Geometry: see drawing. Coordinates: mm, zero at the bounding-box minimum. A direction names the side the tool comes from. Coordinates: 2 decimals unless noted, no trailing zeros. Order: outer loops, then holes, each group sorted by start corner. A loop starts at its lowest first (then second) coordinate and runs counter-clockwise, first axis right, second up.
Item 1: Section A-A on y = 11. Return the cut outline in (x, z), then the cut area to 3 significant figures.
Item 2: Mould query, pull axis Y, two halves, no side actions, for the marked faces 3, 4 and 5. Classes: released by +Y, released by -Y, zero draft, split by the parting line, or undercut.
Item 3: Ray query, line 1 (Y direction, x = 11, z = 0.75); line 2 (Y direction, x = 8.5, z = 0.9); line 3 (X direction, y = 8.25, z = 0.95). Return the intervals inside material, ascending.
Item 4: Contact query for flat-ended pins moving along their axis: P1, Ø2.5, axis at x = 11, y = 9, coming from the +Z side; P2, Ø1.5, axis at x = 14.5, z = 2, coming from the +Y side; P3, Ø1, axis at x = 3.5, z = 4, coming from the +Y side; P4, Ø5, axis at x = 10.5, y = 6.5, coming from the +Z side. Output: stop coordinate, or through.
Item 5: Reachability of the marked faces 1 and 2 from +Z, -Z, +X, -X, +Y, -Y: full face, straight path, thin tool, end or side. Return the list, or none.
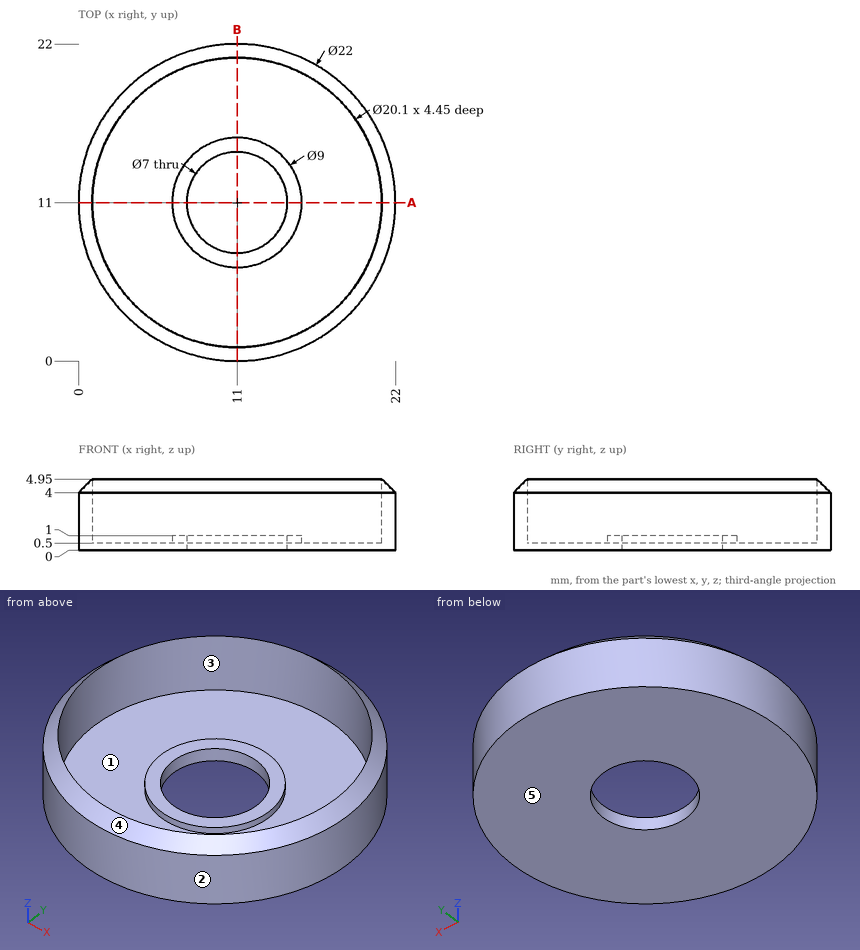
Answer list:
1. outline: (0, 0) - (7.5, 0) - (7.5, 1) - (6.5, 1) - (6.5, 0.5) - (0.95, 0.5) - (0.95, 4.95) - (0, 4) - close; (14.5, 0) - (22, 0) - (22, 4) - (21.05, 4.95) - (21.05, 0.5) - (15.5, 0.5) - (15.5, 1) - (14.5, 1) - close
1. area: 16.1 mm2
2. face 3: undercut
2. face 4: split by the parting line
2. face 5: zero draft
3. line 1: y = 0 to 0.95, 6.5 to 7.5, 14.5 to 15.5, 21.05 to 22
3. line 2: y = 0.29 to 1.27, 7.26 to 8.55, 13.45 to 14.74, 20.73 to 21.71
3. line 3: x = 0.35 to 1.33, 7.44 to 8.83, 13.17 to 14.56, 20.67 to 21.65
4. P1: passes through
4. P2: stops at y = 21.65
4. P3: stops at y = 19.49
4. P4: stops at z = 1
5. face 1: +Z
5. face 2: +Z, -Z
